Geometry: see drawing. Coordinates: mm, zero at the bounding-box minimum. Round coordinates to 2 decimals unless told otherwise and drop trailing zeros. Loops run counter-clockwise (first coordinate to the right, second up) from the corner with the lowest first, then second, coordinate; pieces in that order, holes last.
(1) Material intervals for probe 1 along Y at (x, z) = (2.25, 3.5); probe 2 along Y at (x, z) = (0.85, 6.25); probe 3 along X at (y, z) = (12.5, 3.75), sorted ascending.
(2) Section A-A, the plane x = 2.25. Return the cut outline in (y, z), plus the area to 3 significant figures.
(3) Section D-D, the plane z = 3. Return the cut outline in (x, y).
(4) Section C-C, the plane y = 13.9. Return the cut outline in (x, z).
(5) Mould query, pull axis X, two halves, no side actions, for the marked faces 1, 2, 3 and 4. Classes: pulls with the +X half, pulls with the -X half, needs draft (parallel to the pull), parting line crosses it, or undercut.
(6) Section B-B, the plane z = 5.25. Return the cut outline in (x, y).
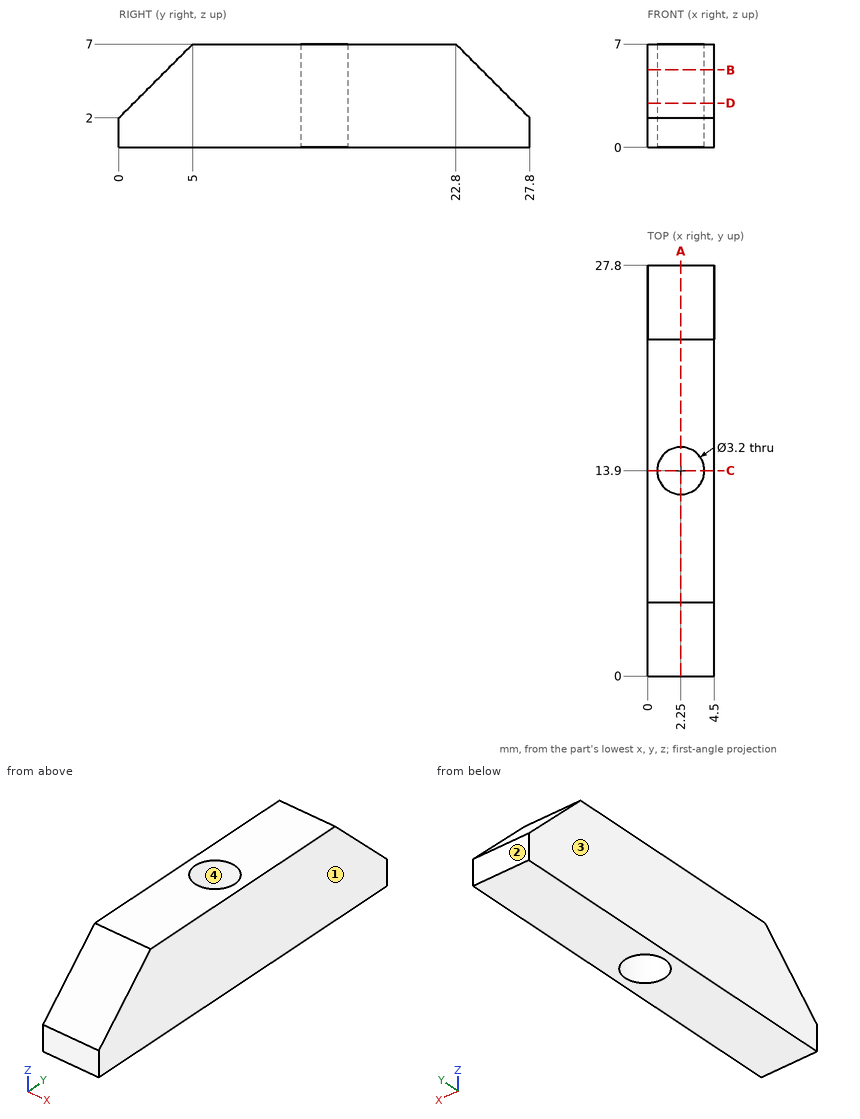
Output values:
1. probe 1: y = 1.5 to 12.3, 15.5 to 26.3
1. probe 2: y = 4.25 to 13.13, 14.67 to 23.55
1. probe 3: x = 0 to 1.48, 3.02 to 4.5
2. outline: (0, 0) - (12.3, 0) - (12.3, 7) - (5, 7) - (0, 2) - close; (15.5, 0) - (27.8, 0) - (27.8, 2) - (22.8, 7) - (15.5, 7) - close
2. area: 147 mm2
3. outline: (0, 1) - (4.5, 1) - (4.5, 26.8) - (0, 26.8) - close; hole circle Ø3.2 at (2.25, 13.9)
4. outline: (0, 0) - (0.65, 0) - (0.65, 7) - (0, 7) - close; (3.85, 0) - (4.5, 0) - (4.5, 7) - (3.85, 7) - close
5. face 1: pulls with the +X half
5. face 2: needs draft
5. face 3: pulls with the -X half
5. face 4: undercut
6. outline: (0, 3.25) - (4.5, 3.25) - (4.5, 24.55) - (0, 24.55) - close; hole circle Ø3.2 at (2.25, 13.9)
